```python
from build123d import *

# Parameters (mm, degrees)
SKETCH_1_W          = 266
SKETCH_1_H          = 126
EXTRUDE_1_DEPTH     = 3
SKETCH_2_W          = 220
SKETCH_2_H          = 19
CUT_EXTRUDE_1_DEPTH = 4
SKETCH_3_W          = 3
SKETCH_3_H          = 19
EXTRUDE_2_DEPTH     = 1
SKETCH_4_W          = 3
SKETCH_4_H          = 19
EXTRUDE_3_DEPTH     = 1
FILLET_1_R          = 3
SKETCH_5_R          = 2.25
CUT_EXTRUDE_2_DEPTH = 4


with BuildPart() as part:
    # Эскиз1 → Бобышка-Вытянуть1 (new body)
    with BuildSketch(Plane(origin=(0, 0, 0), x_dir=(-1, 0, 0), z_dir=(0, 0, -1))):
        with Locations((110, 60)):
            Rectangle(SKETCH_1_W, SKETCH_1_H)
    extrude(amount=EXTRUDE_1_DEPTH)

    # Эскиз2 → Вырез-Вытянуть1 (cut, through all)
    with BuildSketch(Plane.XY):
        with Locations((-110, 90.5)):
            Rectangle(SKETCH_2_W, SKETCH_2_H)
    extrude(amount=-CUT_EXTRUDE_1_DEPTH, mode=Mode.SUBTRACT)

    # Эскиз3 → Бобышка-Вытянуть2 (add)
    with BuildSketch(Plane.ZY):
        with Locations((-1.5, 90.5)):
            Rectangle(SKETCH_3_W, SKETCH_3_H)
    extrude(amount=EXTRUDE_2_DEPTH)

    # Эскиз4 → Бобышка-Вытянуть3 (add)
    with BuildSketch(Plane(origin=(-220, 0, 0), x_dir=(0, 0, -1), z_dir=(1, 0, 0))):
        with Locations((1.5, 90.5)):
            Rectangle(SKETCH_4_W, SKETCH_4_H)
    extrude(amount=EXTRUDE_3_DEPTH)

    # Скругление1
    fillet_1_edges = [part.edges().sort_by_distance(p)[0] for p in [
        (-1, 81, -1.5),
        (-1, 100, -1.5),
        (-219, 100, -1.5),
        (-219, 81, -1.5),
    ]]
    fillet(fillet_1_edges, radius=FILLET_1_R)

    # Эскиз5 → Вырез-Вытянуть2 (cut, through all)
    with BuildSketch(Plane(origin=(0, 0, -3), x_dir=(-1, 0, 0), z_dir=(0, 0, -1))):
        with Locations((230, 110)):
            Circle(SKETCH_5_R)
        with Locations((110, 110)):
            Circle(SKETCH_5_R)
        with Locations((-10, 110)):
            Circle(SKETCH_5_R)
        with Locations((-10, 10)):
            Circle(SKETCH_5_R)
        with Locations((110, 10)):
            Circle(SKETCH_5_R)
        with Locations((230, 10)):
            Circle(SKETCH_5_R)
    extrude(amount=-CUT_EXTRUDE_2_DEPTH, mode=Mode.SUBTRACT)


solid = part.part
```
Work out the finished part from the listing and answer in its coordinate system (mm). Give positions to 0.01 mm unless a question says otherwise; leave off trailing zeros. Loops run counter-clockwise (first coordinate to the right, second up) from the corner with the lowest first, then second, coordinate; pieces in that order, holes last. Notation, with made-up numbers: (-27, 42.5) -> (23, 42.5) arc R20 ccw to (23, 76.5) -> close; hole circle Ø11 at (-35, -26). An arc over 180 degrees is marked (long way). One line per question, with ' | ' between items. Start each with the question number.
1) Determine the mould class of faces 1 (the face through (-112, 59, 0)), 2 (the face through (-112.08, 109.14, -1.52)) for opening direction X: +X half, -X half, draft (parallel to the pull), parting line (faces both ways), or undercut.
2) Straight lines are drawn through the part: L1, parallel to Y at x = 10, z = -1.45; L2, parallel to Y at x = -110, z = -1.7; L3, parallel to Y at x = -186, z = -1.9. For each, find the intervals that lie inside material, in ascending order.
3) Section B-B, the plane z = -1.9 is taken. Determine the outline of the cut face in (x, y), then the cut area to 3 significant figures.
4) Section A-A, the plane x = -48.5 is taken. Determine the outline of the cut face in (y, z), then the cut area to 3 significant figures.
5) This flat-tipped pin is pushed along its axis until it touches: pin 1 (4 mm diameter, centred on x = -230, y = 10, fed in from -Z). Where does it stop, or does it pass through?
Resolved:
1) face 1: draft | face 2: undercut
2) L1: -3 to 7.75, 12.25 to 107.75, 112.25 to 123 | L2: -3 to 7.75, 12.25 to 81, 100 to 107.75, 112.25 to 123 | L3: -3 to 81, 100 to 123
3) outline: (-243, -3) -> (23, -3) -> (23, 123) -> (-243, 123) -> close; hole circle Ø4.5 at (-230, 10); hole circle Ø4.5 at (-230, 110); hole (-219, 84) arc R3 ccw to (-216, 81) -> (-4, 81) arc R3 ccw to (-1, 84) -> (-1, 97) arc R3 ccw to (-4, 100) -> (-216, 100) arc R3 ccw to (-219, 97) -> close; hole circle Ø4.5 at (-110, 10); hole circle Ø4.5 at (-110, 110); hole circle Ø4.5 at (10, 10); hole circle Ø4.5 at (10, 110) | area: 29,300 mm2
4) outline: (-3, -3) -> (81, -3) -> (81, 0) -> (-3, 0) -> close; (100, -3) -> (123, -3) -> (123, 0) -> (100, 0) -> close | area: 321 mm2
5) pin 1: through
